from build123d import *

# Parameters (mm, degrees)
SKETCH1_R           = 2.794
BOSS_EXTRUDE1_DEPTH = 3.937
SKETCH2_R           = 3.81
SKETCH2_R_2         = 2.794
BOSS_EXTRUDE2_DEPTH = 1.27
SKETCH3_R           = 2.794
BOSS_EXTRUDE3_DEPTH = 0.635
SKETCH4_R           = 2.032
BOSS_EXTRUDE4_DEPTH = 15.113
SKETCH5_R           = 2.54
SKETCH5_R_2         = 2.032
BOSS_EXTRUDE5_DEPTH = 0.254
CUT_EXTRUDE1_DEPTH  = 15.24


with BuildPart() as part:
    # Sketch1 → Boss-Extrude1 (new body)
    with BuildSketch(Plane.XY):
        with Locations((7.874, 0)):
            Circle(SKETCH1_R)
        with BuildLine():
            Line((6.35, 0.762), (7.112, 0.762))
            Line((7.112, 0.762), (7.112, 1.524))
            ThreePointArc((7.112, 1.524), (7.874, 2.286), (8.636, 1.524))
            Line((8.636, 1.524), (8.636, 0.762))
            Line((8.636, 0.762), (9.398, 0.762))
            ThreePointArc((9.398, 0.762), (10.16, 0), (9.398, -0.762))
            Line((9.398, -0.762), (8.636, -0.762))
            Line((8.636, -0.762), (8.636, -1.524))
            ThreePointArc((8.636, -1.524), (7.874, -2.286), (7.112, -1.524))
            Line((7.112, -1.524), (7.112, -0.762))
            Line((7.112, -0.762), (6.35, -0.762))
            ThreePointArc((6.35, -0.762), (5.588, 0), (6.35, 0.762))
        make_face(mode=Mode.SUBTRACT)
    boss_extrude1 = extrude(amount=BOSS_EXTRUDE1_DEPTH)

    # Sketch2 → Boss-Extrude2 (add)
    with BuildSketch(Plane(origin=(0, 0, 0), x_dir=(-1, 0, 0), z_dir=(0, 0, -1))):
        with Locations((-7.874, 0)):
            Circle(SKETCH2_R)
        with Locations((-7.874, 0)):
            Circle(SKETCH2_R_2, mode=Mode.SUBTRACT)
    boss_extrude2 = extrude(amount=-BOSS_EXTRUDE2_DEPTH)

    # Mirror1: Boss-Extrude1, Boss-Extrude2 across plane
    add(boss_extrude1.mirror(Plane.XY.offset(3.937)))
    add(boss_extrude2.mirror(Plane.XY.offset(3.937)))

    # Sketch3 → Boss-Extrude3 (add)
    with BuildSketch(Plane.XY.offset(7.874)):
        with Locations((7.874, 0)):
            Circle(SKETCH3_R)
    extrude(amount=BOSS_EXTRUDE3_DEPTH)

    # Sketch4 → Boss-Extrude4 (add)
    with BuildSketch(Plane.XY.offset(8.509)):
        with Locations((7.874, 0)):
            Circle(SKETCH4_R)
    extrude(amount=BOSS_EXTRUDE4_DEPTH)

    # Sketch5 → Boss-Extrude5 (add)
    with BuildSketch(Plane.XY.offset(23.622)):
        with Locations((7.874, 0)):
            Circle(SKETCH5_R)
        with Locations((7.874, 0)):
            Circle(SKETCH5_R_2, mode=Mode.SUBTRACT)
    extrude(amount=-BOSS_EXTRUDE5_DEPTH)

    # Sketch6 → Cut-Extrude1 (cut)
    with BuildSketch(Plane.XY.offset(23.622)):
        with BuildLine():
            Line((8.636, -1.016), (7.112, -1.016))
            ThreePointArc((7.112, -1.016), (6.096, 0), (7.112, 1.016))
            Line((7.112, 1.016), (8.636, 1.016))
            ThreePointArc((8.636, 1.016), (9.652, 0), (8.636, -1.016))
        make_face()
    extrude(amount=-CUT_EXTRUDE1_DEPTH, mode=Mode.SUBTRACT)


solid = part.part
Model file for the job. Use its own axes, mm. A direction names the side the tool comes from. Round coordinates to 2 decimals unless told otherwise and drop trailing zeros. Loops run counter-clockwise (first coordinate to the right, second up) from the corner with the lowest first, then second, coordinate; pieces in that order, holes last. Notation, with made-up numbers: M 13.25,-2 L 27.25,-2 A18 cw 27.25,27 Z; hole C -10.75,87.5 d3. An arc over 180 degrees is marked long. One line per question, with ' | ' between items.
1) Drill centre lines: line 1 along Z through (x, y) = (11, 1.5); line 2 along Y through (x, z) = (8, 9); line 3 along Z through (x, y) = (8, 2.5). Where is each one in solid material? Low to high.
Solved:
line 1: z = 0 to 1.27, 6.6 to 7.87 | line 2: y = -2.03 to -1.02, 1.02 to 2.03 | line 3: z = 0 to 8.51, 23.37 to 23.62
2) Band-saw the part on A-A (z = 12). Give the cut face in (x, y).
Solved:
outline: C 7.87,0 d4.06; hole M 7.11,-1.02 L 8.64,-1.02 A1.02 ccw 8.64,1.02 L 7.11,1.02 A1.02 ccw Z
3) 3-axis set-ups, long thin cutter, end or side, ignore diameter. For faces 1 (the flat face through (9, -1, 0)), 2 (the cylindrical face through (5.083, 0.123, 8.187)), 3 (the flat face through (7, 2, 23.368)): which of +Z, -Z, +X, -X, +Y, -Y reach the whole face in a straight line?
Solved:
face 1: -Z, +X, -X, +Y, -Y | face 2: +Z | face 3: none
4) Flat gauge pins, fed straight in: pin 1 (0.8 mm diameter, centred on y = 1, z = 5, fed in from -X); pin 2 (3 mm diameter, centred on x = 8, z = 11.5, fed in from -Y); pin 3 (0.8 mm diameter, centred on x = 6.5, z = 6.5, fed in from -Y). Where does each tip first touch, or does it go through?
Solved:
pin 1: stops at x = 5.15 | pin 2: stops at y = -2.03 | pin 3: stops at y = -3.68
5) Mould opens along Y. For faces 4 (the cylindrical face through (8.7, -3.72, 7.25)), 5 (the flat face through (9, 3, 6.604)), 6 (the flat face through (8, 0, 7.874)) say: +Y half, -Y half, draft (parallel to the pull), parting line (faces both ways), or undercut.
Solved:
face 4: parting line | face 5: draft | face 6: undercut
6) Band-saw the part on C-C (y = 3.5). Give the cut face in (x, z).
Solved:
outline: M 6.37,0 L 9.38,0 L 9.38,1.27 L 6.37,1.27 Z; M 6.37,6.6 L 9.38,6.6 L 9.38,7.87 L 6.37,7.87 Z
7) Band-saw the part on B-B (x = 11). Give the cut face in (y, z), then the cut area to 3 significant figures.
Solved:
outline: M -2.18,0 L 2.18,0 L 2.18,1.27 L -2.18,1.27 Z; M -2.18,6.6 L 2.18,6.6 L 2.18,7.87 L -2.18,7.87 Z | area: 11.1 mm²
